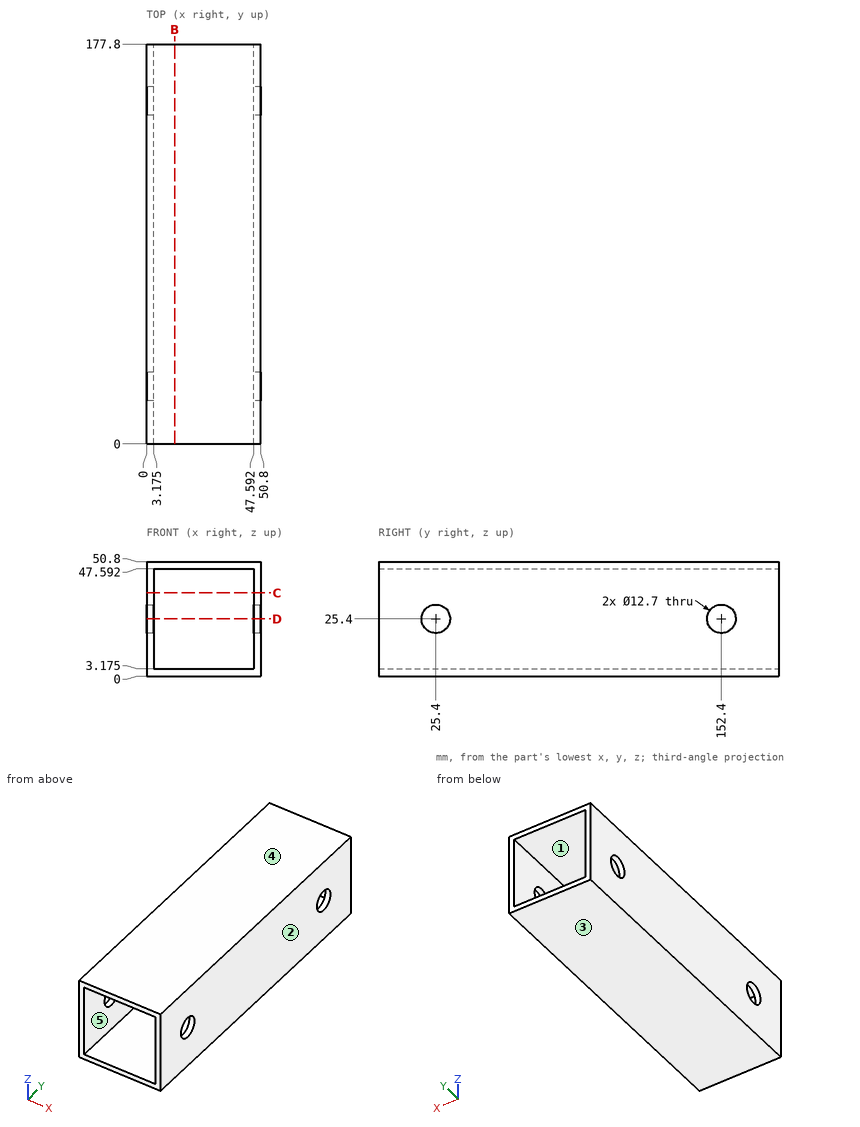
Check sheet for the drawn part. Datum: minimum x, y, z corner. Units: mm. A direction names the side the tool comes from. Round coordinates to 2 decimals unless told otherwise and drop trailing zeros. Order: outer loops, then holes, each group sorted by start corner. A loop starts at its lowest first (then second) coordinate and runs counter-clockwise, first axis right, second up. Notation, with made-up numbers: (-3, 69.5) - (8, 69.5) arc R8 cw to (8, 83.5) - close; hole circle Ø9 at (31, -20). An arc over 180 degrees is marked (long way). Use a Markdown table: item, result. Add a question column.
(1) Sectioned sample at D-D, the plane z = 25.4. Count the separate pieces of the cut face and the enclosed holes in it.
(2) Material ranges on line 1 along Y through (x, z) = (49.55, 25.4); line 2 along X through (y, z) = (142.5, 10) (1 decimal), recorded low to high. Write a range as [from, to].
(3) Sectioned sample at C-C, the plane z = 37. Enter the section's corners in (x, y) (1 decimal), and give its area (4 significant figures).
(4) Tool access check on the marked faces 4 and 5. Record the directions out of +Z, -Z, +X, -X, +Y, -Y that give a thin tool (end or side, any length) a straight path to the whole face; none if there is none.
(5) Depth check by flat-ended pin: pin 1 (10 mm diameter, centred on y = 69, z = 5.5, fed in from -X). Enter the tip coordinate at first touch or a pass-through.
(6) Release check for a two-part mould opening along X. For the marked faces 1, 2 and 3 record: pulls with the +X half, pulls with the -X half, needs draft (parallel to the pull), parting line crosses it, or undercut.
(7) Sectioned sample at B-B, the plane x = 12.5. Enter the section's corners in (y, z) (1 decimal), and give its area (4 significant figures).
Answers below:
| question | item | result |
|---|---|---|
| 1 | separate pieces | 6 |
| 1 | enclosed holes | 0 |
| 2 | line 1 | [0, 19.05], [31.75, 146.05], [158.75, 177.8] |
| 2 | line 2 | [0, 3.2], [47.6, 50.8] |
| 3 | outline | (0, 0) - (3.2, 0) - (3.2, 177.8) - (0, 177.8) - close; (47.6, 0) - (50.8, 0) - (50.8, 177.8) - (47.6, 177.8) - close |
| 3 | area | 1,135 mm² |
| 4 | face 4 | +Z, +X, -X, +Y, -Y |
| 4 | face 5 | +Y, -Y |
| 5 | pin 1 | x = 0 |
| 6 | face 1 | undercut |
| 6 | face 2 | pulls with the +X half |
| 6 | face 3 | needs draft |
| 7 | outline | (0, 0) - (177.8, 0) - (177.8, 3.2) - (0, 3.2) - close; (0, 47.6) - (177.8, 47.6) - (177.8, 50.8) - (0, 50.8) - close |
| 7 | area | 1,135 mm² |
